Can you work these out from the model? Positions are in its coordinate system, mm. A direction names the side the tool comes from. Round coordinates to 2 decimals unless told otherwise and drop trailing zeros. Write each loop counter-clockwise with the first axis right and the second up, starting at its lowest first coordinate (ties: lowest second). Pieces come first, ordered by that corner, then holes. Notation, with made-up numbers: (20, -26.5) -> (71, -26.5) arc R11 cw to (71, -14.5) -> close; hole circle Ø1 at (31, 47). An arc over 180 degrees is marked (long way). Use CSV: the item, a comma, the result in double quotes.
```python
from build123d import *

# Parameters (mm, degrees)
SKETCH_1_R               = 60
SKETCH_1_R_2             = 36
EXTRUDE_1_DEPTH          = 1
CUT_EXTRUDE_1_DEPTH      = 0.5
PATTERN_CIRCULAR_1_COUNT = 12
FILLET_1_R               = 0.5


with BuildPart() as part:
    # Эскиз1 → Бобышка-Вытянуть1 (new, symmetric)
    with BuildSketch(Plane(origin=(0, 0, 0), x_dir=(1, 0, 0), z_dir=(0, 1, 0))):
        with Locations(Location((0, 0, 0), (0, 0, 270))):
            Circle(SKETCH_1_R)
        with Locations(Location((0, 0, 0), (0, 0, 270))):
            Circle(SKETCH_1_R_2, mode=Mode.SUBTRACT)
    extrude(amount=EXTRUDE_1_DEPTH, both=True)

    # Эскиз2 → Вырез-Вытянуть1 (cut)
    with BuildSketch(Plane(origin=(0, 1, 0), x_dir=(1, 0, 0), z_dir=(0, 1, 0))):
        with BuildLine():
            Line((7, 37.5), (-43, 37.5))
            ThreePointArc((-43, 37.5), (-43.5, 38), (-43, 38.5))
            Line((-43, 38.5), (7, 38.5))
            ThreePointArc((7, 38.5), (7.5, 38), (7, 37.5))
        make_face()
    cut_extrude_1 = extrude(amount=-CUT_EXTRUDE_1_DEPTH, mode=Mode.SUBTRACT)

    # Круговой массив1: Вырез-Вытянуть1 ×12 about axis
    pattern_circular_1_axis = Axis((0, 0, 0), (0, 1, 0))
    for i in range(1, PATTERN_CIRCULAR_1_COUNT):
        add(cut_extrude_1.rotate(pattern_circular_1_axis, i * 360 / PATTERN_CIRCULAR_1_COUNT), mode=Mode.SUBTRACT)

    # Скругление1
    fillet_1_edges = [part.edges().sort_by_distance(p)[0] for p in [
        (0, -1, -60),
        (0, 1, -60),
        (0, -1, -36),
        (0, 1, -36),
    ]]
    fillet(fillet_1_edges, radius=FILLET_1_R)


solid = part.part
```
Q1. Will these pins go through, and if not, where does the flat tip stop? P1, Ø12, axis at x = -8, z = -32, coming from the -Y side; P2, Ø0.6, axis at y = 0.5, z = 10, coming from the +X side; P3, Ø0.6, axis at x = -11, y = 0.5, coming from the +Z side; P4, Ø0.8, axis at x = -26.5, z = -38, coming from the +Y side.
Resolved:
P1,"stops at y = -1"
P2,"stops at x = 59.21"
P3,"stops at z = 59.04"
P4,"stops at y = 0.5"
Q2. On a 3-axis mill with a long thin cutter (end or side, diameter ignored), from which of +Z, -Z, +X, -X, +Y, -Y can I reach the whole of each face in a straight line? I mean faces 1 (the face through (10.81, -0.01, 34.34)), 2 (the face through (23.65, 0.75, -34.04)). Say none if no direction works.
Resolved:
face 1,"+Y, -Y"
face 2,"+Y"
Q3. Please list where these lines run through material, in increasing order: probe 1 along X at (y, z) = (0.35, 0); probe 2 along Z at (x, y) = (-25.5, 0.8); probe 3 along X at (y, z) = (0.65, -42.5).
Resolved:
probe 1,"x = -60 to -36, 36 to 60"
probe 2,"z = -54.2 to -38.5, -37.5 to -29.73, -28.58 to -25.55, 25.55 to 29.17, 29.65 to 30.83, 32.83 to 54.2"
probe 3,"x = -42.32 to 1.39, 3.39 to 18.76, 19.92 to 37.5, 38.5 to 42.32"
Q4. Suppose I cut it at B-B (y = 0.15). Write out the boundary of the cut face in (x, z).
Resolved:
outline,"circle Ø120 at (0, 0); hole circle Ø72 at (0, 0)"
Q5. If we mould it in two halves opening along Z, with no side actions, what happens to faces 3 (the face through (2.64, 0.01, -59.94)), 4 (the face through (-24, 0.5, 34))? For each: released by +Z, released by -Z, zero draft, split by the parting line, or undercut.
Resolved:
face 3,"split by the parting line"
face 4,"undercut"
